from build123d import *

# Parameters (mm, degrees)
SKIZZE1_R                       = 2
AUFSATZ_LINEAR_AUSTRAGEN1_DEPTH = 1.5


with BuildPart() as part:
    # Skizze1 → Aufsatz-Linear austragen1 (new, symmetric)
    with BuildSketch(Plane(origin=(0, 0, 0), x_dir=(1, 0, 0), z_dir=(0, 1, 0))):
        Polygon((-2.309401077, 4), (-4.618802154, 0), (-2.309401077, -4), (2.309401077, -4), (4.618802154, 0), (2.309401077, 4), align=None)
        with Locations(Location((0, 0, 0), (0, 0, 270))):
            Circle(SKIZZE1_R, mode=Mode.SUBTRACT)
    extrude(amount=AUFSATZ_LINEAR_AUSTRAGEN1_DEPTH, both=True)

    # Skizze2 → Schnitt-Rotation1 (revolve, cut)
    with BuildSketch(Plane.XY):
        with BuildLine():
            Line((0, 1.5), (0, 2.733189598))
            Line((0, 2.733189598), (4.618802154, 2.733189598))
            Line((4.618802154, 2.733189598), (4.618802154, 1))
            ThreePointArc((4.618802154, 1), (2.405106227, 2.134086305), (0, 1.5))
        make_face()
        with BuildLine():
            Line((4.618802154, -1), (4.618802154, -2.751278334))
            Line((4.618802154, -2.751278334), (0, -2.751278334))
            Line((0, -2.751278334), (0, -1.5))
            ThreePointArc((0, -1.5), (2.428755218, -2.352546333), (4.618802154, -1))
        make_face()
    revolve(axis=Axis((0, 1.5, 0), (0, -1, 0)), mode=Mode.SUBTRACT)


solid = part.part
Work out the finished part from the listing and answer in its coordinate system (mm). Give positions to 0.01 mm unless a question says otherwise; leave off trailing zeros. Loops run counter-clockwise (first coordinate to the right, second up) from the corner with the lowest first, then second, coordinate; pieces in that order, holes last. Notation, with made-up numbers: (25.25, 24) - (41.25, 24) arc R31 cw to (41.25, 61) - close; hole circle Ø6 at (62.5, -10). An arc over 180 degrees is marked (long way). Answer in a Markdown table with one row per item.
(1) Section B-B (y = -0.15) is taken. Give the vertices of the cut face in (x, z).
Results list:
| item | result |
|---|---|
| outline | (-4.62, 0) - (-2.31, -4) - (2.31, -4) - (4.62, 0) - (2.31, 4) - (-2.31, 4) - close; hole circle Ø4 at (0, 0) |
(2) Section C-C (x = 3.5) is taken. Give the vertices of the cut face in (y, z), and give its area (3 significant figures).
Results list:
| item | result |
|---|---|
| outline | (-1.5, -1.94) - (1.5, -1.94) - (1.5, 1.94) - (-1.5, 1.94) - close |
| area | 11.6 mm² |
(3) Consider L1, parallel to X at y = 0.9, z = -1.25; L2, parallel to Z at x = 3, y = 0.85; L3, parallel to X at y = 1.35, z = -1. Determine where each line is inside the solid, lowest interval first. Write a range as [from, to].
Results list:
| item | result |
|---|---|
| L1 | x = [-3.9, -1.56], [1.56, 3.9] |
| L2 | z = [-2.8, 2.8] |
| L3 | x = [-4.04, -1.73], [1.73, 4.04] |
(4) For a pull along X with two mould halves and no side action, classify faces 1 (the face through (-1, -1.5, -2)), 2 (the face through (-2, 0, 0)), 3 (the face through (3.448, 0.021, 2.028)) as pulls with the +X half, pulls with the -X half, needs draft (parallel to the pull), parting line crosses it, or undercut.
Results list:
| item | result |
|---|---|
| face 1 | needs draft |
| face 2 | undercut |
| face 3 | pulls with the +X half |
(5) Section A-A (x = 0) is taken. Give the vertices of the cut face in (y, z), and give its area (3 significant figures).
Results list:
| item | result |
|---|---|
| outline | (-1.5, -4) - (1.5, -4) - (1.5, -2) - (-1.5, -2) - close; (-1.5, 2) - (1.5, 2) - (1.5, 4) - (-1.5, 4) - close |
| area | 12.0 mm² |
